Autodesk Inventor part; units mm, degrees
ref_plane "YZ Plane" through (0, 0, 0) normal (1, 0, 0) x (0, 1, 0)
ref_plane "XZ Plane" through (0, 0, 0) normal (0, 1, 0) x (-1, 0, 0)
ref_plane "XY Plane" through (0, 0, 0) normal (0, 0, 1) x (1, 0, 0)
sketch "Sketch1" plane through (0, 0, 0) normal (0, 1, 0) x (-1, 0, 0)
  line L0 (0, 0) -> (-79.375, 0)
  line L1 (-79.375, 0) -> (-79.375, 38.1)
  line L2 (-79.375, 38.1) -> (0, 38.1)
  line L3 (0, 38.1) -> (0, 0)
  dimension "d0" = 79.375
  dimension "d1" = 38.1
extrude "Extrusion1" add sketch "Sketch1" along normal blind 3.175
sketch "Sketch2" plane through (0, 3.175, 0) normal (0, 1, 0) x (1, 0, 0)
  line L0 (79.375, 0) -> (0, 0)
  line L1 (0, 0) -> (0, -38.1)
  line L2 (0, -38.1) -> (79.375, -38.1)
  line L3 (79.375, -38.1) -> (79.375, 0)
  line L4 (0, -3.175) -> (79.375, -3.175)
  line L5 (79.375, -3.175) -> (79.375, -6.604)
  line L6 (79.375, -6.604) -> (0, -6.604)
  line L7 (0, -6.604) -> (0, -3.175)
  line L8 (79.375, -33.3121) -> (0, -33.3121)
  line L9 (0, -33.3121) -> (0, -36.5125)
  line L10 (0, -36.5125) -> (79.375, -36.5125)
  line L11 (79.375, -36.5125) -> (79.375, -33.3121)
  dimension "d4" = 3.429
  dimension "d5" = 3.175
  dimension "d6" = 3.2004
  dimension "d7" = 1.5875
extrude "Extrusion2" cut sketch "Sketch2" against normal blind 1.5875 contours L3 L6 L1 L4 | L3 L10 L1 L8
properties part number "Electronics Container Part 3"
Geometry: final body of the model. Coordinates: model frame, mm. A direction names the side the tool comes from. Give positions to 0.01 mm unless a question says otherwise; leave off trailing zeros. Order: outer loops, then holes, each group sorted by start corner. A loop starts at its lowest first (then second) coordinate and runs counter-clockwise, first axis right, second up. Notation, with made-up numbers: M -18,-29 L -6,-29 A36 ccw -6,8 Z; hole C -26,57.5 d2. An arc over 180 degrees is marked long. Answer as CSV lines item,"result". Start each with the question number.
1) First-contact query: P1, Ø1, axis at x = 27.5, z = 4.5, coming from the +Y side. Flat tip, straight axial feed; report the tip coordinate or a pass-through.
2) Cut plane A-A (x = 36.5). Output: boundary loops of the cut face in (y, z) (1 decimal), then the cut area to 3 significant figures.
3) Line query: line 1 (Z direction, x = 52, y = 2.4) (1 decimal); line 2 (Y direction, x = 29, z = 4.5). Output: solid intervals per line, ascending. Write a range as from..to.
4) Set-up query: faces 1 (the flat face through (40, 2, 33.312)), 2 (the flat face through (40, 3.175, 37)). Return all of +Z, -Z, +X, -X, +Y, -Y with unobstructed straight access to the full face (end or side cutting, diameter ignored); none if empty.
5) Cut plane B-B (z = 4.5). Output: boundary loops of the cut face in (x, y) (1 decimal), then the cut area to 3 significant figures.
6) Mould query, pull axis Z, two halves, no side actions, for faces 3 (the flat face through (39, 2, 36.512)), 4 (the flat face through (40, 3.175, 2)), 5 (the flat face through (39, 2, 0)). Classes: +Z half, -Z half, draft (parallel to the pull), parting line (faces both ways), or undercut.
Findings below:
1,P1,"stops at y = 1.59"
2,outline,"M 0,0 L 3.2,0 L 3.2,3.2 L 1.6,3.2 L 1.6,6.6 L 3.2,6.6 L 3.2,33.3 L 1.6,33.3 L 1.6,36.5 L 3.2,36.5 L 3.2,38.1 L 0,38.1 Z"
2,area,"110 mm²"
3,line 1,"z = 0..3.2, 6.6..33.3, 36.5..38.1"
3,line 2,"y = 0..1.59"
4,face 1,"+X, -X, +Y"
4,face 2,"+Z, -Z, +X, -X, +Y"
5,outline,"M 0,0 L 79.4,0 L 79.4,1.6 L 0,1.6 Z"
5,area,"126 mm²"
6,face 3,"undercut"
6,face 4,"draft"
6,face 5,"-Z half"
